The listing builds one solid part. Answer for the finished solid, in the listing's coordinates (mm). A direction names the side the tool comes from. Round coordinates to 2 decimals unless told otherwise and drop trailing zeros. Write each loop counter-clockwise with the first axis right and the second up, starting at its lowest first coordinate (ties: lowest second). Pieces come first, ordered by that corner, then holes.
Item 1: A tool of negligible diameter and unlimited length cuts with its end or side. For faces 5 (the face through (22.225, -3, 1)), 6 (the face through (0, -13, 57.15)), 7 (the face through (-22.225, -2, 1)), 8 (the face through (0.34, -9.52, 0.8)), 9 (the face through (5.556, 12, 1)), from which of +Z, -Z, +X, -X, +Y, -Y can it reach the whole face along a straight path? Write none if from no direction.
Item 2: For a pull along X with two mould halves and no side action, classify faces 1 (the face through (19.88, 13.46, 0.8)), 2 (the face through (-5.556, 12, 1)), 3 (the face through (28.654, -19.788, 46.817)), 4 (the face through (12, 15.875, 1)) as +X half, -X half, draft (parallel to the pull), parting line (faces both ways), or undercut.
Item 3: Find section A-A on z = 44.45. Give the number of separate pieces and of enclosed holes in the cut face, then the cut area to 3 significant figures.
Item 4: Find the intervals of material crossed by probe 1 along X at (y, z) = (-19, 44) (3 decimals); probe 2 along Y at (x, z) = (-24, -19.5) (1 decimal); probe 3 along X at (y, z) = (14, -31), in increasing order.
Item 5: Each of these flat-tipped pins is pushed along its axis until it touches: pin 1 (9 mm diameter, centred on y = 13.5, z = -18.5, fed in from -X) (3 decimals); pin 2 (9 mm diameter, centred on x = -30.16, z = 44.45, fed in from +Y) (3 decimals); pin 3 (2 mm diameter, centred on y = 10.5, z = -43.5, fed in from +X) (3 decimals); pin 4 (17 mm diameter, centred on x = 0, y = 0, fed in from -Z). Where does it stop, or does it pass through?
Item 6: Find section B-B on y = 0. Give the vertices of the cut face in (x, z) (3 decimals), then the cut area to 3 significant figures.
```python
from build123d import *

# Parameters (mm, degrees)
EXTRUDE1_DEPTH         = 57.15
F_10_CLEARANCE_HOLE1_D = 5.6134
CHAMFER1_SIZE          = 4.7625


with BuildPart() as part:
    # Sketch1 → Extrude1 (new, symmetric)
    with BuildSketch(Plane.XY):
        with BuildLine():
            Line((22.225, 15.875), (5.55625, 15.875))
            Line((5.55625, 15.875), (5.55625, 7.736518011))
            ThreePointArc((5.55625, 7.736518011), (0, -9.525), (-5.55625, 7.736518011))
            Line((-5.55625, 7.736518011), (-5.55625, 15.875))
            Line((-5.55625, 15.875), (-22.225, 15.875))
            Line((-22.225, 15.875), (-22.225, -15.875))
            Line((-22.225, -15.875), (-34.925, -15.875))
            Line((-34.925, -15.875), (-34.925, -23.8125))
            Line((-34.925, -23.8125), (34.925, -23.8125))
            Line((34.925, -23.8125), (34.925, -15.875))
            Line((34.925, -15.875), (22.225, -15.875))
            Line((22.225, -15.875), (22.225, 15.875))
        make_face()
    extrude(amount=EXTRUDE1_DEPTH, both=True)

    # #10 Clearance Hole1 (through all)
    with Locations(Plane.XZ.offset(23.8125)):
        with Locations((-30.1625, -44.45), (30.1625, -44.45), (-30.1625, 44.45), (30.1625, 44.45)):
            Hole(F_10_CLEARANCE_HOLE1_D / 2)

    # Chamfer1
    chamfer1_edges = [part.edges().sort_by_distance(p)[0] for p in [
        (-22.225, 15.875, 0),
        (22.225, 15.875, 0),
    ]]
    chamfer(chamfer1_edges, length=CHAMFER1_SIZE)


solid = part.part
```
Check values:
1. face 5: +Z, -Z, +X, +Y
1. face 6: +Z, +X, -X, +Y, -Y
1. face 7: +Z, -Z, -X, +Y
1. face 8: +Z, -Z
1. face 9: +Z, -Z, +Y
2. face 1: +X half
2. face 2: undercut
2. face 3: undercut
2. face 4: draft
3. separate pieces: 3
3. enclosed holes: 0
3. area: 1,490 mm2
4. probe 1: x = -34.925 to -32.933, -27.392 to 27.392, 32.933 to 34.925
4. probe 2: y = -23.8 to -15.9
4. probe 3: x = -19.34 to -5.56, 5.56 to 19.34
5. pin 1: stops at x = -22.225
5. pin 2: stops at y = -15.875
5. pin 3: stops at x = 22.225
5. pin 4: passes through
6. outline: (-22.225, -57.15) - (-9.525, -57.15) - (-9.525, 57.15) - (-22.225, 57.15) - close; (9.525, -57.15) - (22.225, -57.15) - (22.225, 57.15) - (9.525, 57.15) - close
6. area: 2,900 mm2
